Could you check a few things on this drawing? It's one solid part, dimensions in mm from its lowest x, y, z. Coordinates: 2 decimals unless noted, no trailing zeros. Order: outer loops, then holes, each group sorted by start corner. A loop starts at its lowest first (then second) coordinate and runs counter-clockwise, first axis right, second up.
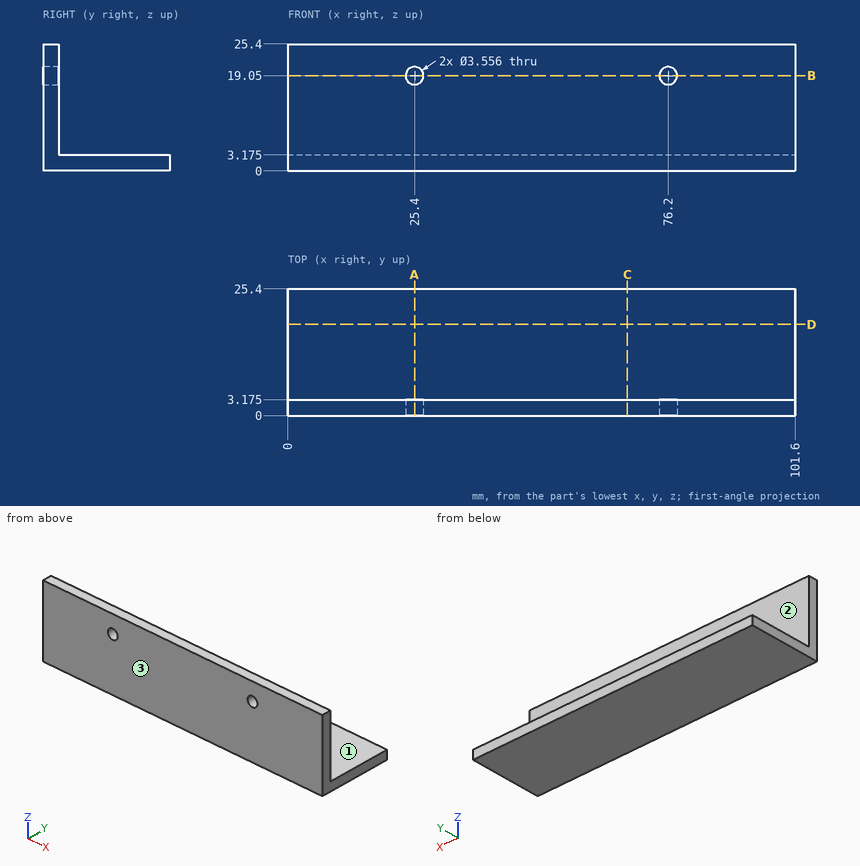
1. I'm going to push flat-ended pins straight in: pin 1 (3 mm diameter, centred on x = 76.2, z = 19.05, fed in from -Y) (3 decimals); pin 2 (6.5 mm diameter, centred on x = 72, z = 14.5, fed in from +Y) (3 decimals). Where does each tip first touch, or does it pass through?
Completed:
pin 1: passes through
pin 2: stops at y = 3.175
2. Imagine slicing it at C-C on x = 68. Please give me the cut outline in (y, z) (3 decimals), then the cut area to 3 significant figures.
Completed:
outline: (0, 0) - (25.4, 0) - (25.4, 3.175) - (3.175, 3.175) - (3.175, 25.4) - (0, 25.4) - close
area: 151 mm2
3. Imagine slicing it at A-A on x = 25.4. Please give me the cut outline in (y, z) (3 decimals).
Completed:
outline: (0, 0) - (25.4, 0) - (25.4, 3.175) - (3.175, 3.175) - (3.175, 17.272) - (0, 17.272) - close; (0, 20.828) - (3.175, 20.828) - (3.175, 25.4) - (0, 25.4) - close
4. Imagine slicing it at D-D on y = 18.25. Please give me the cut outline in (x, z) (3 decimals), then the cut area to 3 significant figures.
Completed:
outline: (0, 0) - (101.6, 0) - (101.6, 3.175) - (0, 3.175) - close
area: 323 mm2
5. Imagine slicing it at B-B on z = 19.05. Please give me the cut outline in (x, y) (3 decimals).
Completed:
outline: (0, 0) - (23.622, 0) - (23.622, 3.175) - (0, 3.175) - close; (27.178, 0) - (74.422, 0) - (74.422, 3.175) - (27.178, 3.175) - close; (77.978, 0) - (101.6, 0) - (101.6, 3.175) - (77.978, 3.175) - close
6. Thinking about a two-plate mould opening in Y: for the marked faces 1, 2 and 3, which applies, pulls with the +Y half, pulls with the -Y half, needs draft (parallel to the pull), parting line crosses it, or undercut?
Completed:
face 1: needs draft
face 2: pulls with the +Y half
face 3: pulls with the -Y half
7. Please list where these lines run through material, in increasing order: probe 1 along X at (y, z) = (2.4, 19.05); probe 2 along Z at (x, y) = (76.2, 1.7); probe 3 along Y at (x, z) = (37.5, 5) (3 decimals).
Completed:
probe 1: x = 0 to 23.62, 27.18 to 74.42, 77.98 to 101.6
probe 2: z = 0 to 17.27, 20.83 to 25.4
probe 3: y = 0 to 3.175
